```python
from build123d import *

# Parameters (mm, degrees)
F1_DEPTH = 6.35
F2_R     = 6.35


with BuildPart() as f1:
    # F0 (on Top) → F1 (new body)
    with BuildSketch(Plane.XY):
        with BuildLine():
            add(Edge.make_bspline(
                [(-19.8501589651, 15.875), (-20.3419955534, 15.232168206), (-20.8064619249, 14.5688414833)],
                knots=[1.5189156006, 1.5189156006, 1.5189156006, 1.5707963268, 1.5707963268, 1.5707963268], degree=2, weights=[1, 0.9996635676, 1]))
            ThreePointArc((-20.8064619249, 14.5688414833), (-25.386887881, -0.8160414938), (-19.8278686449, -15.875))
            ThreePointArc((-19.8278686449, -15.875), (0.8160414938, -25.386887881), (20.8064619249, -14.5688414833))
            add(Edge.make_bspline(
                [(20.8064619249, -14.5688414833), (25.5490601214, -7.7957093222), (26.9403423198, 0)],
                knots=[4.7123889804, 4.7123889804, 4.7123889804, 5.2303546369, 5.2303546369, 5.2303546369], degree=2, weights=[1, 0.9666509732, 1]))
            add(Edge.make_bspline(
                [(26.9403423198, 0), (29.9920251657, 17.099358015), (17.9011443111, 25.5654838108)],
                knots=[5.2303546369, 5.2303546369, 5.2303546369, 6.2831853127, 6.2831853127, 6.2831853127], degree=2, weights=[1, 0.8646136894, 1]))
            add(Edge.make_bspline(
                [(17.9011443111, 25.5654838108), (-1.8529265857, 39.3974329633), (-19.8501589651, 15.875)],
                knots=[5.5e-09, 5.5e-09, 5.5e-09, 1.5189156006, 1.5189156006, 1.5189156006], degree=2, weights=[1, 0.7252094391, 1]))
        make_face()
        with BuildLine():
            ThreePointArc((-19.8278686449, -15.875), (-25.386887881, -0.8160414938), (-20.8064619249, 14.5688414833))
            add(Edge.make_bspline(
                [(-19.8501589651, 15.875), (-20.3419955534, 15.232168206), (-20.8064619249, 14.5688414833)],
                knots=[1.5189156006, 1.5189156006, 1.5189156006, 1.5707963268, 1.5707963268, 1.5707963268], degree=2, weights=[1, 0.9996635676, 1]))
            Line((-19.8501589651, 15.875), (-121.4278686449, 15.875))
            Line((-121.4278686449, 15.875), (-121.4278686449, -15.875))
            Line((-121.4278686449, -15.875), (-19.8278686449, -15.875))
        make_face()
    extrude(amount=F1_DEPTH)

    # F2
    f2_edges = [f1.edges().sort_by_distance(p)[0] for p in [
        (-121.427869, 15.875, 3.175),
        (-121.427869, -15.875, 3.175),
    ]]
    fillet(f2_edges, radius=F2_R)


solid = f1.part
```
For this review, take the finished solid that the model builds, in its own axes (mm). A direction names the side the tool comes from. Give positions to 0.01 mm unless a question says otherwise; leave off trailing zeros. Write each loop counter-clockwise with the first axis right and the second up, starting at its lowest first coordinate (ties: lowest second). Pieces come first, ordered by that corner, then holes.
Item 1: Take a section at A-A (x = -40). Give the boundary of the cut face in (y, z) (3 decimals), and give its area (3 significant figures).
Item 2: Insertion check: P1, Ø1, axis at y = 14.5, z = 3, coming from the +X side; P2, Ø3, axis at x = -48, z = 3.5, coming from the +Y side (3 decimals); P3, Ø3, axis at y = -5.5, z = 1, coming from the +X side. Each pin has a flat end and moves straight along its axis. Give the tip position at first contact, or say it passes through.
Item 3: Wall thickness on probe 1 along Y at (x, z) = (-101, 5.5) (3 decimals); probe 2 along X at (y, z) = (4.5, 3.75); probe 3 along X at (y, z) = (-19.5, 1): over which ranges is each line inside the solid? List them lowest first.
Item 4: Take a section at B-B (y = -21). Give the boundary of the cut face in (x, z), and give its area (3 significant figures).
Item 5: Machinability: for faces 1 (the face through (-67, 15.875, 3)), 2 (the face through (0.486, -25.395, 3.131)), 3 (the face through (-68, -15.875, 3)), which of the approach directions +Z, -Z, +X, -X, +Y, -Y give a long, thin tool a straight path to every point of the face, cutting with its end or side? Answer none if there is none.
Established:
1. outline: (-15.875, 0) - (15.875, 0) - (15.875, 6.35) - (-15.875, 6.35) - close
1. area: 202 mm2
2. P1: stops at x = 26.19
2. P2: stops at y = 15.875
2. P3: stops at x = 25.98
3. probe 1: y = -15.875 to 15.875
3. probe 2: x = -121.43 to 27.43
3. probe 3: x = -16.28 to 16.28
4. outline: (-14.29, 0) - (14.29, 0) - (14.29, 6.35) - (-14.29, 6.35) - close
4. area: 181 mm2
5. face 1: +Z, -Z, -X, +Y
5. face 2: +Z, -Z, -Y
5. face 3: +Z, -Z, -X, -Y
